The listing builds one solid part. Answer for the finished solid, in the listing's coordinates (mm). A direction names the side the tool comes from. Give positions to 0.01 mm unless a question says otherwise; leave off trailing zeros. Order: outer loops, then holes, each group sorted by start corner. A loop starts at its lowest first (then second) coordinate and runs counter-clockwise, first axis right, second up. Notation, with made-up numbers: (36, -14) - (59, -14) arc R10 ccw to (59, -8) - close; hole circle Ø8 at (-15, 89). An arc over 180 degrees is marked (long way). Answer as a JSON object with one key per item and string values. Group by question number.
Q1. Consider line 1 (Y direction, x = 84, z = 0.6); line 2 (X direction, y = -19.5, z = 3.75); line 3 (Y direction, x = 76.2, z = 1.35) (3 decimals). Determine where each line is inside the solid, lowest interval first.
Q2. The mould has two halves that part along X. Classify faces 6 (the face through (-15.24, 100, 3)), 7 (the face through (88, 57.912, 3)), 8 (the face through (-100.7, 54.07, 2.63)): released by +X, released by -X, zero draft, split by the parting line, or undercut.
Q3. A cutting plane is placed at C-C, the plane x = 86.5. Give the vertices of the cut face in (y, z), and give its area (3 significant figures).
Q4. A cutting plane is placed at B-B, the plane y = 90.5. Give the vertices of the cut face in (x, z), and give its area (3 significant figures).
Q5. For faces 1 (the face through (2.413, -101, 3)), 2 (the face through (8.93, 113.95, 2.63)), 3 (the face through (-93, 37.338, 3)), 4 (the face through (101.6, -41, 3)), 5 (the face through (15.24, 100, 3)), determine the directions among +Z, -Z, +X, -X, +Y, -Y from which every point of the face is accessible in a straight line to the end or side of a thin tool.
Q6. Given pin 1 (5 mm diameter, centred on x = 45, y = -40.5, fed in from -Z); pin 2 (1.2 mm diameter, centred on x = -100.5, z = 2.5, fed in from +Y); pin 3 (1.5 mm diameter, centred on x = 64, z = 4.5, fed in from -Y); pin 4 (1.6 mm diameter, centred on y = 106.5, z = 4, fed in from -X), each flat-ended and moving along its own axis, determine where each tip first touches the part or whether it passes through.
Q7. A cutting plane is placed at A-A, the plane x = -50.8. Give the vertices of the cut face in (y, z) (3 decimals).
Q8. A cutting plane is placed at D-D, the plane y = -78.74. Give the vertices of the cut face in (x, z) (3 decimals).
from build123d import *

# Parameters (mm, degrees)
SKETCH1_R           = 114.3
BOSS_EXTRUDE1_DEPTH = 5.334
TOPBOTTOMCUTS_DEPTH = 162.732592745
SIDECUTS_DEPTH      = 162.714591138
SKETCH4_W           = 2.4638
SKETCH4_H           = 19.05
SKETCH4_W_2         = 5.334
MOTORMOUNTS_DEPTH   = 162.714591138
SKETCH5_R           = 3.175
BOLTHOLES_DEPTH     = 162.714591138
SKETCH6_W           = 22.352
SKETCH6_H           = 83.470360746
WHEEL_CUTOUTS_DEPTH = 162.714591138


with BuildPart() as part:
    # Sketch1 → Boss-Extrude1 (new body)
    with BuildSketch(Plane.XY):
        Circle(SKETCH1_R)
        with BuildLine():
            Line((-40.299999918, 49.073006904), (-40.299999918, -49.073006904))
            ThreePointArc((-40.299999918, -49.073006904), (0, -63.5), (40.299999918, -49.073006904))
            Line((40.299999918, -49.073006904), (40.299999918, 49.073006904))
            ThreePointArc((40.299999918, 49.073006904), (0, 63.5), (-40.299999918, 49.073006904))
        make_face(mode=Mode.SUBTRACT)
    extrude(amount=BOSS_EXTRUDE1_DEPTH)

    # Sketch2 → TopBottomCuts (cut, through all)
    with BuildSketch(Plane.XY.offset(5.334)):
        Polygon((-20.066, 92.964), (-20.066, 116.329451538), (-15.24, 116.329451538), (-15.24, 92.964), (-15.24, 86.614), (-20.066, 86.614), align=None)
        Polygon((15.24, 92.964), (15.24, 86.614), (20.066, 86.614), (20.066, 92.964), (20.066, 116.329451538), (15.24, 116.329451538), align=None)
        Polygon((-2.413, 92.964), (-2.413, 86.614), (2.413, 86.614), (2.413, 92.964), (2.413, 116.329451538), (-2.413, 116.329451538), align=None)
        Polygon((20.066, -116.329451538), (20.066, -92.964), (20.066, -86.614), (15.24, -86.614), (15.24, -92.964), (15.24, -116.329451538), align=None)
        Polygon((2.413, -116.329451538), (2.413, -92.964), (2.413, -86.614), (-2.413, -86.614), (-2.413, -92.964), (-2.413, -116.329451538), align=None)
        Polygon((-15.24, -116.329451538), (-15.24, -92.964), (-15.24, -86.614), (-20.066, -86.614), (-20.066, -92.964), (-20.066, -116.329451538), align=None)
    extrude(amount=-TOPBOTTOMCUTS_DEPTH, mode=Mode.SUBTRACT)

    # Sketch3 → SideCuts (cut, through all)
    with BuildSketch(Plane.XY.offset(5.334)):
        Polygon((-83.82, 37.338), (-77.47, 37.338), (-77.47, 32.512), (-83.82, 32.512), (-110.947890819, 32.512), (-110.947890819, 37.338), align=None)
        Polygon((-83.82, 62.738), (-104.163602824, 62.738), (-104.163602824, 57.912), (-83.82, 57.912), (-77.47, 57.912), (-77.47, 62.738), align=None)
        Polygon((-83.82, 50.038), (-77.47, 50.038), (-77.47, 45.212), (-83.82, 45.212), (-108.296559878, 45.212), (-108.296559878, 50.038), align=None)
        Polygon((110.947890819, 32.512), (83.82, 32.512), (77.47, 32.512), (77.47, 37.338), (83.82, 37.338), (110.947890819, 37.338), align=None)
        Polygon((108.296559878, 45.212), (83.82, 45.212), (77.47, 45.212), (77.47, 50.038), (83.82, 50.038), (108.296559878, 50.038), align=None)
        Polygon((77.47, 62.738), (77.47, 57.912), (83.82, 57.912), (104.163602824, 57.912), (104.163602824, 62.738), (83.82, 62.738), align=None)
    extrude(amount=-SIDECUTS_DEPTH, mode=Mode.SUBTRACT)

    # Sketch4 → MotorMounts (cut, through all)
    with BuildSketch(Plane.XY.offset(5.334)):
        with Locations((-100.3681, -41.275)):
            Rectangle(SKETCH4_W, SKETCH4_H)
        with Locations((-100.3681, 0)):
            Rectangle(SKETCH4_W, SKETCH4_H)
        with Locations((-78.469199932, 0)):
            Rectangle(SKETCH4_W_2, SKETCH4_H)
        with Locations((-42.966999918, 0)):
            Rectangle(SKETCH4_W_2, SKETCH4_H)
        with Locations((-78.469199932, -41.275)):
            Rectangle(SKETCH4_W_2, SKETCH4_H)
        with Locations((-42.966999918, -41.275)):
            Rectangle(SKETCH4_W_2, SKETCH4_H)
        with Locations((42.966999918, -41.275)):
            Rectangle(SKETCH4_W_2, SKETCH4_H)
        with Locations((78.469199932, -41.275)):
            Rectangle(SKETCH4_W_2, SKETCH4_H)
        with Locations((100.3681, -41.275)):
            Rectangle(SKETCH4_W, SKETCH4_H)
        with Locations((42.966999918, 0)):
            Rectangle(SKETCH4_W_2, SKETCH4_H)
        with Locations((78.469199932, 0)):
            Rectangle(SKETCH4_W_2, SKETCH4_H)
        with Locations((100.3681, 0)):
            Rectangle(SKETCH4_W, SKETCH4_H)
    extrude(amount=-MOTORMOUNTS_DEPTH, mode=Mode.SUBTRACT)

    # Sketch5 → BoltHoles (cut, through all)
    with BuildSketch(Plane.XY.offset(5.334)):
        with Locations((-76.2, -78.74)):
            Circle(SKETCH5_R)
        with Locations((-50.8, 78.74)):
            Circle(SKETCH5_R)
        with Locations(Location((76.2, -78.74, 0), (0, 0, 180))):
            Circle(SKETCH5_R)
        with Locations(Location((50.8, 78.74, 0), (0, 0, 180))):
            Circle(SKETCH5_R)
    extrude(amount=-BOLTHOLES_DEPTH, mode=Mode.SUBTRACT)

    # Sketch6 → Wheel Cutouts (cut, through all)
    with BuildSketch(Plane.XY.offset(5.334)):
        with Locations((-114.3, -7.559146116)):
            Rectangle(SKETCH6_W, SKETCH6_H)
        with Locations((114.3, -7.559146116)):
            Rectangle(SKETCH6_W, SKETCH6_H)
    extrude(amount=-WHEEL_CUTOUTS_DEPTH, mode=Mode.SUBTRACT)


solid = part.part
Reply:
{
 "1": {"line 1": "y = -77.51 to 32.51, 37.34 to 45.21, 50.04 to 57.91, 62.74 to 77.51", "line 2": "x = -103.12 to -40.3, 40.3 to 103.12", "line 3": "y = -85.194 to -81.915, -75.565 to -50.8, -31.75 to -9.525, 9.525 to 85.194"},
 "2": {"face 6": "undercut", "face 7": "zero draft", "face 8": "released by -X"},
 "3": {"outline": "(-74.71, 0) - (32.51, 0) - (32.51, 5.33) - (-74.71, 5.33) - close; (37.34, 0) - (45.21, 0) - (45.21, 5.33) - (37.34, 5.33) - close; (50.04, 0) - (57.91, 0) - (57.91, 5.33) - (50.04, 5.33) - close; (62.74, 0) - (74.71, 0) - (74.71, 5.33) - (62.74, 5.33) - close", "area": "720 mm^2"},
 "4": {"outline": "(-69.82, 0) - (-20.07, 0) - (-20.07, 5.33) - (-69.82, 5.33) - close; (-15.24, 0) - (-2.41, 0) - (-2.41, 5.33) - (-15.24, 5.33) - close; (2.41, 0) - (15.24, 0) - (15.24, 5.33) - (2.41, 5.33) - close; (20.07, 0) - (69.82, 0) - (69.82, 5.33) - (20.07, 5.33) - close", "area": "668 mm^2"},
 "5": {"face 1": "+Z, -Z, -Y", "face 2": "+Z, -Z, +X, +Y", "face 3": "+Z, -Z, -X", "face 4": "+Z, -Z", "face 5": "+Z, -Z, +Y"},
 "6": {"pin 1": "stops at z = 0", "pin 2": "stops at y = 55.54", "pin 3": "stops at y = -95.2", "pin 4": "stops at x = -43.5"},
 "7": {"outline": "(-102.391, 0) - (75.565, 0) - (75.565, 5.334) - (-102.391, 5.334) - close; (81.915, 0) - (102.391, 0) - (102.391, 5.334) - (81.915, 5.334) - close"},
 "8": {"outline": "(-82.852, 0) - (-79.375, 0) - (-79.375, 5.334) - (-82.852, 5.334) - close; (-73.025, 0) - (73.025, 0) - (73.025, 5.334) - (-73.025, 5.334) - close; (79.375, 0) - (82.852, 0) - (82.852, 5.334) - (79.375, 5.334) - close"}
}
